from build123d import *

# Parameters (mm, degrees)
BOSS_EXTRU_1_DEPTH      = 2.1
ESQUISSE2_R             = 2.2499999999999973
BOSS_EXTRU_2_DEPTH      = 0.2
ENL_V_START             = -0.8
ESQUISSE4_R             = 2.2499999999999973
ENL_V_MAT_EXTRU_1_DEPTH = 0.8
BOSS_EXTRU_3_START      = 2.5
ESQUISSE5_R             = 3.349999999999999
ESQUISSE5_R_2           = 2.2499999999999973
BOSS_EXTRU_3_DEPTH      = 4.8
ESQUISSE6_R             = 2.2499999999999973
ESQUISSE6_R_2           = 1.1
ENL_V_MAT_EXTRU_2_DEPTH = 3.1
ENL_V_MAT_EXTRU_3_REACH = 14.163
ESQUISSE7_R             = 0.4999999999999999
ESQUISSE7_R_2           = 0.5000000000000001
ESQUISSE7_R_3           = 0.5000000000000003
ESQUISSE7_R_4           = 0.49999999999999895


with BuildPart() as part:
    # Esquisse1 → Boss.-Extru.1 (new body)
    with BuildSketch(Plane(origin=(0, 0, 0), x_dir=(1, 0, 0), z_dir=(0, 1, 0))):
        with BuildLine():
            Line((-6.770489387338948, 3.2903216238761672), (-7.3999999999999995, 3.349999999999998))
            ThreePointArc((-7.3999999999999995, 3.349999999999998), (-9.76880771697493, 2.368807716974932), (-10.749999999999995, 1.67e-15))
            Line((-10.75, 1.97e-15), (-8.499999999999998, 1.97e-15))
            ThreePointArc((-8.499999999999998, 2.11e-15), (-7.399999999999999, 1.100000000000002), (-6.299999999999999, 1.97e-15))
            Line((-6.299999999999999, 1.97e-15), (10.75, 1.97e-15))
            ThreePointArc((10.75, 2.03e-15), (10.222792206135784, 1.2727922061357861), (8.95, 1.8000000000000005))
            Line((8.95, 1.8000000000000007), (-6.770489387338948, 3.2903216238761672))
        make_face()
        with BuildLine():
            Line((-8.499999999999998, 1.97e-15), (-10.75, 1.97e-15))
            ThreePointArc((-10.749999999999995, 1.67e-15), (-9.76880771697493, -2.3688077169749304), (-7.3999999999999995, -3.349999999999998))
            Line((-7.3999999999999995, -3.349999999999998), (-6.770489387338948, -3.2903216238761672))
            Line((-6.770489387338948, -3.2903216238761672), (8.95, -1.799999999999998))
            ThreePointArc((8.949999999999998, -1.7999999999999992), (10.222792206135784, -1.272792206135785), (10.75, 2.03e-15))
            Line((10.75, 1.97e-15), (-6.299999999999999, 1.97e-15))
            ThreePointArc((-6.299999999999999, 1.71e-15), (-7.399999999999999, -1.099999999999998), (-8.499999999999998, 2.11e-15))
        make_face()
    extrude(amount=BOSS_EXTRU_1_DEPTH)

    # Esquisse2 → Boss.-Extru.2 (add)
    # profile 1 of 3: a face of its own
    with BuildSketch(Plane(origin=(0, 2.1, 0), x_dir=(1, 0, 0), z_dir=(0, 1, 0))):
        with BuildLine():
            Line((-6.770489387338715, 3.290321623876145), (-7.399999999999999, 3.3499999999999974))
            ThreePointArc((-7.3999999999999995, 3.3499999999999974), (-10.749999999999995, 1.8e-16), (-7.4, -3.3499999999999983))
            Line((-7.3999999999999995, -3.349999999999998), (-6.770489387338895, -3.2903216238761623))
            ThreePointArc((-6.770489387338895, -3.290321623876155), (-4.8182021232855305, -2.1346708701325934), (-4.050000000000001, 1.15e-15))
            ThreePointArc((-4.050000000000001, 1.97e-15), (-4.818202123285472, 2.1346708701325254), (-6.770489387338716, 3.290321623876124))
        make_face()
        with Locations(Location((-7.399999999999999, 1.97e-15, 0), (0, 0, 270))):
            Circle(ESQUISSE2_R, mode=Mode.SUBTRACT)
    # profile 2 of 3: a face of its own
    with BuildSketch(Plane(origin=(0, 2.1, 0), x_dir=(1, 0, 0), z_dir=(0, 1, 0))):
        with BuildLine():
            ThreePointArc((-6.770489387338715, 3.290321623876124), (-7.083833461594222, 3.3350470341499694), (-7.3999999999999995, 3.3499999999999996))
            Line((-7.399999999999999, 3.3499999999999974), (-6.770489387338715, 3.290321623876145))
        make_face()
    # profile 3 of 3: a face of its own
    with BuildSketch(Plane(origin=(0, 2.1, 0), x_dir=(1, 0, 0), z_dir=(0, 1, 0))):
        with BuildLine():
            Line((-6.770489387338895, -3.2903216238761623), (-7.3999999999999995, -3.349999999999998))
            ThreePointArc((-7.3999999999999995, -3.349999999999996), (-7.0838334615943115, -3.3350470341499743), (-6.770489387338895, -3.290321623876155))
        make_face()
    extrude(amount=BOSS_EXTRU_2_DEPTH)

    # Esquisse4 → Enlèv. mat.-Extru.1 (cut)
    with BuildSketch(Plane(origin=(0, 2.3000000000000003, 0), x_dir=(1, 0, 0), z_dir=(0, 1, 0)).offset(ENL_V_START)):
        with Locations(Location((-7.399999999999999, 1.97e-15, 0), (0, 0, 270))):
            Circle(ESQUISSE4_R)
    extrude(amount=ENL_V_MAT_EXTRU_1_DEPTH, mode=Mode.SUBTRACT)

    # Esquisse5 → Boss.-Extru.3 (add)
    with BuildSketch(Plane.XZ.offset(BOSS_EXTRU_3_START)):
        with Locations(Location((-7.399999999999999, -1.97e-15, 0), (0, 0, 90))):
            Circle(ESQUISSE5_R)
        with Locations(Location((-7.399999999999999, -1.97e-15, 0), (0, 0, 90))):
            Circle(ESQUISSE5_R_2, mode=Mode.SUBTRACT)
    extrude(amount=-BOSS_EXTRU_3_DEPTH)

    # Esquisse6 → Enlèv. mat.-Extru.2 (cut)
    with BuildSketch(Plane.XZ.offset(2.499999999999999)):
        with Locations(Location((-7.399999999999999, -1.97e-15, 0), (0, 0, 90))):
            Circle(ESQUISSE6_R)
        with Locations(Location((-7.399999999999999, -1.97e-15, 0), (0, 0, 270))):
            Circle(ESQUISSE6_R_2, mode=Mode.SUBTRACT)
    extrude(amount=-ENL_V_MAT_EXTRU_2_DEPTH, mode=Mode.SUBTRACT)

    # Esquisse7 → Enlèv. mat.-Extru.3 (cut, up to next)
    with BuildSketch(Plane(origin=(0, 2.1, 0), x_dir=(1, 0, 0), z_dir=(0, 1, 0)), mode=Mode.PRIVATE) as enl_v_mat_extru_3_sk1:
        with Locations(Location((-2.55, -3e-17, 0), (0, 0, 270))):
            Circle(ESQUISSE7_R)
    enl_v_mat_extru_3_tool1 = extrude(enl_v_mat_extru_3_sk1.sketch, amount=-ENL_V_MAT_EXTRU_3_REACH, mode=Mode.PRIVATE) & part.part
    # Esquisse7 → Enlèv. mat.-Extru.3 (cut, up to next)
    with BuildSketch(Plane(origin=(0, 2.1, 0), x_dir=(1, 0, 0), z_dir=(0, 1, 0)), mode=Mode.PRIVATE) as enl_v_mat_extru_3_sk2:
        with Locations(Location((-0.7500000000000002, -1e-17, 0), (0, 0, 270))):
            Circle(ESQUISSE7_R_2)
    enl_v_mat_extru_3_tool2 = extrude(enl_v_mat_extru_3_sk2.sketch, amount=-ENL_V_MAT_EXTRU_3_REACH, mode=Mode.PRIVATE) & part.part
    # Esquisse7 → Enlèv. mat.-Extru.3 (cut, up to next)
    with BuildSketch(Plane(origin=(0, 2.1, 0), x_dir=(1, 0, 0), z_dir=(0, 1, 0)), mode=Mode.PRIVATE) as enl_v_mat_extru_3_sk3:
        with Locations(Location((1.0499999999999994, 1e-17, 0), (0, 0, 270))):
            Circle(ESQUISSE7_R_3)
    enl_v_mat_extru_3_tool3 = extrude(enl_v_mat_extru_3_sk3.sketch, amount=-ENL_V_MAT_EXTRU_3_REACH, mode=Mode.PRIVATE) & part.part
    # Esquisse7 → Enlèv. mat.-Extru.3 (cut, up to next)
    with BuildSketch(Plane(origin=(0, 2.1, 0), x_dir=(1, 0, 0), z_dir=(0, 1, 0)), mode=Mode.PRIVATE) as enl_v_mat_extru_3_sk4:
        with Locations(Location((2.8499999999999988, 2e-17, 0), (0, 0, 270))):
            Circle(ESQUISSE7_R_3)
    enl_v_mat_extru_3_tool4 = extrude(enl_v_mat_extru_3_sk4.sketch, amount=-ENL_V_MAT_EXTRU_3_REACH, mode=Mode.PRIVATE) & part.part
    # Esquisse7 → Enlèv. mat.-Extru.3 (cut, up to next)
    with BuildSketch(Plane(origin=(0, 2.1, 0), x_dir=(1, 0, 0), z_dir=(0, 1, 0)), mode=Mode.PRIVATE) as enl_v_mat_extru_3_sk5:
        with Locations(Location((4.649999999999998, 4e-17, 0), (0, 0, 270))):
            Circle(ESQUISSE7_R)
    enl_v_mat_extru_3_tool5 = extrude(enl_v_mat_extru_3_sk5.sketch, amount=-ENL_V_MAT_EXTRU_3_REACH, mode=Mode.PRIVATE) & part.part
    # Esquisse7 → Enlèv. mat.-Extru.3 (cut, up to next)
    with BuildSketch(Plane(origin=(0, 2.1, 0), x_dir=(1, 0, 0), z_dir=(0, 1, 0)), mode=Mode.PRIVATE) as enl_v_mat_extru_3_sk6:
        with Locations(Location((6.4499999999999975, 6e-17, 0), (0, 0, 270))):
            Circle(ESQUISSE7_R_4)
    enl_v_mat_extru_3_tool6 = extrude(enl_v_mat_extru_3_sk6.sketch, amount=-ENL_V_MAT_EXTRU_3_REACH, mode=Mode.PRIVATE) & part.part
    # Esquisse7 → Enlèv. mat.-Extru.3 (cut, up to next)
    with BuildSketch(Plane(origin=(0, 2.1, 0), x_dir=(1, 0, 0), z_dir=(0, 1, 0)), mode=Mode.PRIVATE) as enl_v_mat_extru_3_sk7:
        with Locations(Location((8.249999999999996, 8e-17, 0), (0, 0, 270))):
            Circle(ESQUISSE7_R_4)
    enl_v_mat_extru_3_tool7 = extrude(enl_v_mat_extru_3_sk7.sketch, amount=-ENL_V_MAT_EXTRU_3_REACH, mode=Mode.PRIVATE) & part.part
    add(enl_v_mat_extru_3_tool1.solids().sort_by_distance((-2.55, 2.1, 0))[0], mode=Mode.SUBTRACT)
    add(enl_v_mat_extru_3_tool2.solids().sort_by_distance((-0.75, 2.1, 0))[0], mode=Mode.SUBTRACT)
    add(enl_v_mat_extru_3_tool3.solids().sort_by_distance((1.05, 2.1, 0))[0], mode=Mode.SUBTRACT)
    add(enl_v_mat_extru_3_tool4.solids().sort_by_distance((2.85, 2.1, 0))[0], mode=Mode.SUBTRACT)
    add(enl_v_mat_extru_3_tool5.solids().sort_by_distance((4.65, 2.1, 0))[0], mode=Mode.SUBTRACT)
    add(enl_v_mat_extru_3_tool6.solids().sort_by_distance((6.45, 2.1, 0))[0], mode=Mode.SUBTRACT)
    add(enl_v_mat_extru_3_tool7.solids().sort_by_distance((8.25, 2.1, 0))[0], mode=Mode.SUBTRACT)


solid = part.part
Can you work these out from the model? Positions are in its coordinate system, mm. A direction names the side the tool comes from. Coordinates: 2 decimals unless noted, no trailing zeros. Order: outer loops, then holes, each group sorted by start corner. A loop starts at its lowest first (then second) coordinate and runs counter-clockwise, first axis right, second up. Notation, with made-up numbers: (1, -11.75) -> (40, -11.75) arc R32 ccw to (40, 22.25) -> close; hole circle Ø11 at (38, 41). An arc over 180 degrees is marked (long way). Use one line per item in the form item = value.
Q1. Which directions (+Z, -Z, +X, -X, +Y, -Y) give clear straight access to the entire face, cutting with the end or side of a thin tool? Please do faces 1 (the face through (-6, 0.6, -1)), 2 (the face through (-3.038, 1.065, -0.108)), 3 (the face through (-9.596, 1.894, -0.488)).
From the geometry:
face_1 = -Y
face_2 = +Y, -Y
face_3 = +Y
Q2. We'd pull the mould along Z, two halves only. Please class faces 4 (the face through (-10.72, -0.67, -0.44)), 5 (the face through (-5, -2.5, 1)), 6 (the face through (0.562, 1.065, -0.108)): released by +Z, released by -Z, zero draft, split by the parting line, or undercut.
From the geometry:
face_4 = split by the parting line
face_5 = zero draft
face_6 = undercut
Q3. Imagine slicing it at C-C, the plane y = -0.2. List the corners of the cut face in (x, z) for me.
From the geometry:
outline = circle Ø6.7 at (-7.4, 0); hole circle Ø4.5 at (-7.4, 0)
Q4. Will these pins go through, and if not, where does the flat tip stop? P1, Ø1.3, axis at x = 2.85, z = 0, coming from the -Y side; P2, Ø1.6, axis at x = 1.05, z = 0, coming from the +Y side; P3, Ø1.5, axis at x = -4, y = -1, coming from the -Z side.
From the geometry:
P1 = 0
P2 = 2.1
P3 = -2.05
Q5. Imagine slicing it at A-A, the plane z = 0.75. List the corners of the cut face in (x, y) for me.
From the geometry:
outline = (-10.66, -2.5) -> (-9.52, -2.5) -> (-9.52, 0.6) -> (-8.2, 0.6) -> (-8.2, 1.5) -> (-9.52, 1.5) -> (-9.52, 2.3) -> (-10.66, 2.3) -> close; (-6.6, 0.6) -> (-5.28, 0.6) -> (-5.28, -2.5) -> (-4.14, -2.5) -> (-4.14, 0) -> (10.59, 0) -> (10.59, 2.1) -> (-4.14, 2.1) -> (-4.14, 2.3) -> (-5.28, 2.3) -> (-5.28, 1.5) -> (-6.6, 1.5) -> close
Q6. Imagine slicing it at D-D, the plane x = 1.05. List the corners of the cut face in (y, z) for me, then the cut area to 3 significant figures.
From the geometry:
outline = (0, -2.55) -> (2.1, -2.55) -> (2.1, -0.5) -> (0, -0.5) -> close; (0, 0.5) -> (2.1, 0.5) -> (2.1, 2.55) -> (0, 2.55) -> close
area = 8.61 mm²
Q7. Imagine slicing it at B-B, the plane x = 4.65. List the corners of the cut face in (y, z) for me, then the cut area to 3 significant figures.
From the geometry:
outline = (0, -2.21) -> (2.1, -2.21) -> (2.1, -0.5) -> (0, -0.5) -> close; (0, 0.5) -> (2.1, 0.5) -> (2.1, 2.21) -> (0, 2.21) -> close
area = 7.17 mm²
Q8. I need wall thicknesses on L1, parallel to X at y = -0.9, z = 0; L2, parallel to Y at x = -2.75, z = 1; L3, parallel to Z at x = 1.25, y = 1.45. Which ranges of each line are inside material? Lowest first, please.
From the geometry:
L1 = -10.75 to -9.65, -5.15 to -4.05
L2 = 0 to 2.1
L3 = -2.53 to -0.46, 0.46 to 2.53
